For this review, take the finished solid that the model builds, in its own axes (mm). Round coordinates to 2 decimals unless told otherwise and drop trailing zeros. Order: outer loops, then holes, each group sorted by start corner. A loop starts at its lowest first (then second) coordinate and runs counter-clockwise, first axis right, second up. Notation, with made-up numbers: (81.5, 28) - (92.5, 28) arc R30 ccw to (92.5, 63) - close; hole circle Ø6 at (45.25, 55). An arc over 180 degrees is marked (long way). One line per question, with ' | ' between items.
```python
from build123d import *

# Parameters (mm, degrees)
F0_W     = 600
F0_H     = 300
F1_DEPTH = 25
F2_R     = 5
F4_DEPTH = 10
F6_DEPTH = 25


with BuildPart() as f1:
    # F0 (on Front) → F1 (new body)
    with BuildSketch(Plane.XZ):
        Rectangle(F0_W, F0_H)
    extrude(amount=-F1_DEPTH)

    # F2
    f2_edges = [f1.edges().sort_by_distance(p)[0] for p in [
        (300, 12.5, -150),
        (-300, 12.5, -150),
        (300, 12.5, 150),
        (-300, 12.5, 150),
    ]]
    fillet(f2_edges, radius=F2_R)

    # F3 (on face) → F4 (cut)
    with BuildSketch(Plane.XZ):
        with BuildLine():
            Line((-70, -100), (70, -100))
            ThreePointArc((70, -100), (73.535534, -98.535534), (75, -95))
            Line((75, -95), (75, -5))
            ThreePointArc((75, -5), (73.535534, -1.464466), (70, 0))
            Line((70, 0), (-70, 0))
            ThreePointArc((-70, 0), (-73.535534, -1.464466), (-75, -5))
            Line((-75, -5), (-75, -95))
            ThreePointArc((-75, -95), (-73.535534, -98.535534), (-70, -100))
        make_face()
    extrude(amount=-F4_DEPTH, mode=Mode.SUBTRACT)

    # F5 (on face) → F6 (cut)
    with BuildSketch(Plane.XZ.offset(-10)):
        with BuildLine():
            Line((60, -10), (-60, -10))
            ThreePointArc((-60, -10), (-63.535534, -11.464466), (-65, -15))
            Line((-65, -15), (-65, -85))
            ThreePointArc((-65, -85), (-63.535534, -88.535534), (-60, -90))
            Line((-60, -90), (60, -90))
            ThreePointArc((60, -90), (63.535534, -88.535534), (65, -85))
            Line((65, -85), (65, -15))
            ThreePointArc((65, -15), (63.535534, -11.464466), (60, -10))
        make_face()
    extrude(amount=-F6_DEPTH, mode=Mode.SUBTRACT)


solid = f1.part
```
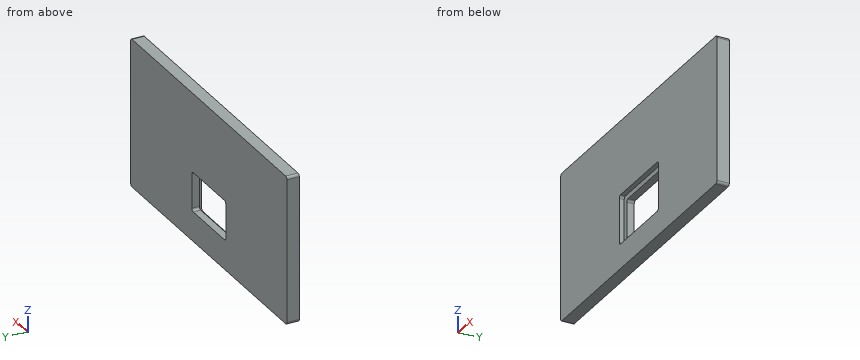
(1) We need section C-C on y = 13.75. State the section outline as (x, z) points.
Output values:
outline: (-300, -145) arc R5 ccw to (-295, -150) - (295, -150) arc R5 ccw to (300, -145) - (300, 145) arc R5 ccw to (295, 150) - (-295, 150) arc R5 ccw to (-300, 145) - close; hole (-65, -85) arc R5 ccw to (-60, -90) - (60, -90) arc R5 ccw to (65, -85) - (65, -15) arc R5 ccw to (60, -10) - (-60, -10) arc R5 ccw to (-65, -15) - close
(2) We need section B-B on x = -53. State the section outline as (y, z) points, plus the area to 3 significant figures.
Output values:
outline: (0, -150) - (25, -150) - (25, -90) - (10, -90) - (10, -100) - (0, -100) - close; (0, 0) - (10, 0) - (10, -10) - (25, -10) - (25, 150) - (0, 150) - close | area: 5,300 mm^2
(3) We need section A-A on z = -27. State the section outline as (x, y) points.
Output values:
outline: (-300, 0) - (-75, 0) - (-75, 10) - (-65, 10) - (-65, 25) - (-300, 25) - close; (65, 10) - (75, 10) - (75, 0) - (300, 0) - (300, 25) - (65, 25) - close
(4) For probe 1 along Z at (x, y) = (42, 15.25); probe 2 along Z at (x, y) = (-18, 8); probe 3 along X at (y, z) = (18, -23), list the stretches that pass through material, from the lowest coordinate up. Write a range as [from, to].
Output values:
probe 1: [-150, -90], [-10, 150] | probe 2: [-150, -100], [0, 150] | probe 3: [-300, -65], [65, 300]
